Build history of the part. All positions in model axes, mm. A direction names the side the tool comes from. Give positions to 0.01 mm unless a question says otherwise; leave off trailing zeros. Order: outer loops, then holes, each group sorted by start corner. A loop starts at its lowest first (then second) coordinate and runs counter-clockwise, first axis right, second up. Notation, with made-up numbers: M 17.5,-12 L 47.5,-12 A35 ccw 47.5,25 Z; hole C 39.25,15 d6. An arc over 180 degrees is marked long. One line per item, written item: value. Start each with the question number.
from build123d import *

# Parameters (mm, degrees)
SKETCH2_R           = 2
BOSS_EXTRUDE1_DEPTH = 20


with BuildPart() as part:
    # Sketch1 → Revolve1 (revolve)
    with BuildSketch(Plane.XY):
        Polygon((0, 0), (0, -12), (10, -12), (10, -2), (1.25, -2), (1.25, 0), align=None)
    revolve(axis=Axis((0, 0, 0), (0, 1, 0)))

    # Sketch2 → Boss-Extrude1 (add)
    with BuildSketch(Plane.XY):
        with Locations((0, -7)):
            Circle(SKETCH2_R)
    extrude(amount=BOSS_EXTRUDE1_DEPTH)


solid = part.part
1) Slice it at D-D (z = 12). List the corners of the cut face in (x, y).
2) Tool access for faces 1 (the flat face through (0, -7, 20)), 2 (the cylindrical face through (-0.27, -0.99, 1.22)), 3 (the cylindrical face through (1.908, -6.399, 14.825)): list every direction of +Z, -Z, +X, -X, +Y, -Y with a clear straight run to the whole face (end or side of a thin tool).
3) Drop flat-ended pins along their axis: P1, Ø2, axis at x = -2, y = -1.5, coming from the -Z side; P2, Ø1, axis at x = 3.5, y = -2, coming from the -Z side; P3, Ø6, axis at x = -6.5, y = -3, coming from the -Z side. Give the stop position or say it passes through.
4) Drill centre lines: line 1 (Y direction, x = -5.25, z = 3); line 2 (X direction, y = -5.75, z = 6); line 3 (Z direction, x = 1.5, y = -7). Where is each one in solid material? Low to high.
5) Slice it at B-B (x = 0). List the corners of the cut face in (y, z), plus the area to 3 significant figures.
6) Slice it at C-C (y = -4). List the corners of the cut face in (x, z).
7) Slice it at A-A (z = 0). List the corners of the cut face in (x, y).
Results list:
1. outline: C 0,-7 d4
2. face 1: +Z, +X, -X, +Y, -Y
2. face 2: +Y
2. face 3: +Z
3. P1: stops at z = -9.94
3. P2: stops at z = -9.54
3. P3: stops at z = -9.37
4. line 1: y = -12 to -2
4. line 2: x = -8 to 8
4. line 3: z = -9.89 to 20
5. outline: M -12,-10 L -2,-10 L -2,-1.25 L 0,-1.25 L 0,1.25 L -2,1.25 L -2,10 L -5,10 L -5,20 L -9,20 L -9,10 L -12,10 Z
5. area: 245 mm²
6. outline: C 0,0 d20
7. outline: M -10,-12 L 10,-12 L 10,-2 L 1.25,-2 L 1.25,0 L -1.25,0 L -1.25,-2 L -10,-2 Z
